from build123d import *

# Parameters (mm, degrees)
SKETCH_1_W          = 95
SKETCH_1_H          = 53
EXTRUDE_282_DEPTH   = 1.2
EXTRUDE_686_DEPTH   = 35
SKETCH_10_W         = 25
SKETCH_10_H         = 25
CUT_EXTRUDE_1_DEPTH = 8
SKETCH_7_R          = 4.5
EXTRUDE_1043_DEPTH  = 42
HOLE_WIZARD_M5_1_D  = 5.3


with BuildPart() as part:
    # 草图1 → Extrude 282 (new body)
    with BuildSketch(Plane(origin=(0, 0, 0), x_dir=(1, 0, 0), z_dir=(0, 1, 0))):
        Rectangle(SKETCH_1_W, SKETCH_1_H)
    extrude(amount=EXTRUDE_282_DEPTH)

    # 草图6 → Extrude 686 (add)
    with BuildSketch(Plane.XZ):
        Polygon((32.5, -56.5), (7.5, -56.5), (7.5, -31.5), (-32.5, -31.5), (-32.5, 31.5), (32.5, 31.5), align=None)
    extrude(amount=EXTRUDE_686_DEPTH)

    # 草图10 → 切除-拉伸1 (cut)
    with BuildSketch(Plane(origin=(0, 0, 0), x_dir=(1, 0, 0), z_dir=(0, 1, 0))):
        with Locations((20, 44)):
            Rectangle(SKETCH_10_W, SKETCH_10_H)
    extrude(amount=-CUT_EXTRUDE_1_DEPTH, mode=Mode.SUBTRACT)

    # 草图7 → Extrude 1043 (add)
    with BuildSketch(Plane(origin=(0, 1.2, 0), x_dir=(1, 0, 0), z_dir=(0, 1, 0))):
        with Locations(Location((0, 0, 0), (0, 0, 90))):
            Circle(SKETCH_7_R)
    extrude(amount=EXTRUDE_1043_DEPTH)

    # M5 间隙孔1 (through all)
    with Locations(Plane(origin=(0, 1.2, 0), x_dir=(1, 0, 0), z_dir=(0, 1, 0))):
        with Locations((-41.25, 20.4), (-41.25, -20.1), (41.35, -20.1), (41.35, 20.4)):
            Hole(HOLE_WIZARD_M5_1_D / 2)


solid = part.part
Geometry check sheet. Reference: the model listing, model coordinates, mm. A direction names the side the tool comes from. Give positions to 0.01 mm unless a question says otherwise; leave off trailing zeros. Order: outer loops, then holes, each group sorted by start corner. A loop starts at its lowest first (then second) coordinate and runs counter-clockwise, first axis right, second up. Notation, with made-up numbers: M -23.75,81.5 L -13.75,81.5 A12 cw -13.75,86.5 Z; hole C -7.5,15.5 d11. An arc over 180 degrees is marked long. Use a Markdown table: item, result.
Item 1: Section check C-C (z = 0). Record the cut outline in (x, y), and give its area (3 significant figures).
Answers follow:
| item | result |
|---|---|
| outline | M -47.5,0 L -32.5,0 L -32.5,-35 L 32.5,-35 L 32.5,0 L 47.5,0 L 47.5,1.2 L 4.5,1.2 L 4.5,43.2 L -4.5,43.2 L -4.5,1.2 L -47.5,1.2 Z |
| area | 2,770 mm2 |
Item 2: Depth check by flat-ended pin: P1, Ø7, axis at x = -41.25, z = 20.1, coming from the -Y side; P2, Ø3, axis at x = 17.5, z = -19.5, coming from the +Y side; P3, Ø10.5, axis at y = -13, z = 3.5, coming from the -X side; P4, Ø5, axis at x = 41.35, z = -20.4, coming from the -Y side. Enter the tip coordinate at first touch or a pass-through.
Answers follow:
| item | result |
|---|---|
| P1 | stops at y = 0 |
| P2 | stops at y = 1.2 |
| P3 | stops at x = -32.5 |
| P4 | passes through |
Item 3: Tool access check on faces 4 (the flat face through (0, 0, 29)), 5 (the flat face through (0, 0, -29)), 6 (the cylindrical face through (-1.352, 21.906, -4.292)). Record the directions out of +Z, -Z, +X, -X, +Y, -Y that give a thin tool (end or side, any length) a straight path to the whole face; none if there is none.
Answers follow:
| item | result |
|---|---|
| face 4 | +Z, +X, -X, +Y |
| face 5 | -Z, +X, -X, +Y |
| face 6 | +Y |
Item 4: Section check B-B (z = -20.4). Record the cut outline in (x, y), and give its area (3 significant figures).
Answers follow:
| item | result |
|---|---|
| outline | M -47.5,0 L -43.9,0 L -43.9,1.2 L -47.5,1.2 Z; M -38.6,0 L -32.5,0 L -32.5,-35 L 32.5,-35 L 32.5,0 L 38.7,0 L 38.7,1.2 L -38.6,1.2 Z; M 44,0 L 47.5,0 L 47.5,1.2 L 44,1.2 Z |
| area | 2,380 mm2 |
Item 5: Draft check along Z on faces 1 (the cylindrical face through (-38.6, 0.6, 20)), 2 (the flat face through (20, -21, -56.5)), 3 (the flat face through (20, -8, -44)). Enter one of: +Z half, -Z half, draft (parallel to the pull), parting line (faces both ways), or undercut.
Answers follow:
| item | result |
|---|---|
| face 1 | undercut |
| face 2 | -Z half |
| face 3 | draft |
Item 6: Material ranges on line 1 along Z through (x, y) = (41.35, 0.4); line 2 along X through (y, z) = (0.5, -20.4); line 3 along Y through (x, z) = (30.5, 20), recorded low to high.
Answers follow:
| item | result |
|---|---|
| line 1 | z = -26.5 to -23.05, -17.75 to 17.45, 22.75 to 26.5 |
| line 2 | x = -47.5 to -43.9, -38.6 to 38.7, 44 to 47.5 |
| line 3 | y = -35 to 1.2 |
Item 7: Section check D-D (x = -18). Record the cut outline in (y, z), and give its area (3 significant figures).
Answers follow:
| item | result |
|---|---|
| outline | M -35,-31.5 L 0,-31.5 L 0,-26.5 L 1.2,-26.5 L 1.2,26.5 L 0,26.5 L 0,31.5 L -35,31.5 Z |
| area | 2,270 mm2 |
Item 8: Section check A-A (x = 41.35). Record the cut outline in (y, z).
Answers follow:
| item | result |
|---|---|
| outline | M 0,-26.5 L 1.2,-26.5 L 1.2,-23.05 L 0,-23.05 Z; M 0,-17.75 L 1.2,-17.75 L 1.2,17.45 L 0,17.45 Z; M 0,22.75 L 1.2,22.75 L 1.2,26.5 L 0,26.5 Z |
